Autodesk Inventor part; units mm, degrees
ref_plane "YZ Plane" through (0, 0, 0) normal (1, 0, 0) x (0, 1, 0)
ref_plane "XZ Plane" through (0, 0, 0) normal (0, 1, 0) x (-1, 0, 0)
ref_plane "XY Plane" through (0, 0, 0) normal (0, 0, 1) x (1, 0, 0)
sketch "Sketch1" plane through (0, 0, 0) normal (0, 0, 1) x (1, 0, 0)
  circle A0 centre (0, 0) radius 1.65
  circle A1 centre (0, 0) radius 2.5
  dimension "d0" = 3.3
  dimension "d1" = 5
extrude "Extrusion1" add sketch "Sketch1" along normal blind 5
sketch "Sketch2" plane through (0, 0, 0) normal (0, 0, 1) x (1, 0, 0)
  circle A0 centre (0, 0) radius 2.5
extrude "Extrusion2" add sketch "Sketch2" against normal blind 1
sketch "Sketch3" plane through (0, 0, -1) normal (0, 0, -1) x (-1, 0, 0)
  circle A0 centre (0, 0) radius 1.6
  dimension "d6" = 3.2
extrude "Extrusion3" add sketch "Sketch3" along normal blind 4
fillet "Fillet1" radius 1 2 edges at (-2.5, 0, -1) (-2.5, 0, 5)
properties part number "Hat"
Design review of the part built by this model. Coordinates are the model's own, in mm. Give positions to 0.01 mm unless a question says otherwise; leave off trailing zeros. Write each loop counter-clockwise with the first axis right and the second up, starting at its lowest first coordinate (ties: lowest second). Pieces come first, ordered by that corner, then holes.
(1) Add section D-D (z = -1.5). Give the boundary of the cut face in (x, y).
Checked values:
outline: circle Ø3.2 at (0, 0)
(2) Add section C-C (z = 0.25). Give the boundary of the cut face in (x, y).
Checked values:
outline: circle Ø5 at (0, 0); hole circle Ø3.3 at (0, 0)
(3) Wall thickness on line 1 along Y through (x, z) = (0, 3.2); line 2 along Y through (x, z) = (0.5, 4.5); line 3 along X through (y, z) = (0.1, -3): over which ranges is each line inside the solid? List them lowest first.
Checked values:
line 1: y = -2.5 to -1.65, 1.65 to 2.5
line 2: y = -2.32 to -1.57, 1.57 to 2.32
line 3: x = -1.6 to 1.6
(4) Mouldability with a two-part tool opening along Y and no side actions: class faces 1 (the face through (0, 0, 0)), 2 (the face through (1.27, 0.97, -2.97)), 3 (the face through (0, 0, -5)), 4 (the face through (-1.216, -1.115, 2.465)) as +Y half, -Y half, draft (parallel to the pull), parting line (faces both ways), or undercut.
Checked values:
face 1: undercut
face 2: parting line
face 3: draft
face 4: undercut
(5) Clearance check with a flat-ended pin moving along its axis: pin 1 Ø1 at (x, y) = (0.5, 0) entering from +Z. State where the tip first meets the part, or that it passes through.
Checked values:
pin 1: stops at z = 0
(6) Add section A-A (x = 0). Give the boundary of the cut face in (y, z), and give its area (3 significant figures).
Checked values:
outline: (-2.5, -0.01) arc R1 ccw to (-1.6, -1) - (-1.6, -5) - (1.6, -5) - (1.6, -1) arc R1 ccw to (2.5, -0.01) - (2.5, 4.01) arc R1 ccw to (1.65, 5) - (1.65, 0) - (-1.65, 0) - (-1.65, 5) arc R1 ccw to (-2.5, 4.01) - close
area: 25.5 mm2
